The listing builds one solid part. Answer for the finished solid, in the listing's coordinates (mm). Face numbers are marked on the shaded views. A direction names the side the tool comes from. Coordinates: 2 decimals unless noted, no trailing zeros. Loops run counter-clockwise (first coordinate to the right, second up) from the corner with the lowest first, then second, coordinate; pieces in that order, holes last. Notation, with made-up numbers: (51, 24.25) -> (66, 24.25) arc R24 cw to (66, 53.25) -> close; hole circle Ø10 at (62, -1.75). An arc over 180 degrees is marked (long way). Answer in a Markdown table with one row per item.
Autodesk Inventor part; units mm, degrees
ref_plane "YZ Plane" through (0, 0, 0) normal (1, 0, 0) x (0, 1, 0)
ref_plane "XZ Plane" through (0, 0, 0) normal (0, 1, 0) x (-1, 0, 0)
ref_plane "XY Plane" through (0, 0, 0) normal (0, 0, 1) x (1, 0, 0)
sketch "Sketch1" plane through (0, 0, 0) normal (0, 0, 1) x (1, 0, 0)
  line L0 (4.1434, -12.66) -> (3.2904, -12.66)
  line L1 (-14.9, 12.8) -> (14.9, 12.8)
  line L2 (14.9, 12.8) -> (14.9, -12.8)
  line L3 (14.9, -12.8) -> (-14.9, -12.8)
  line L4 (-14.9, -12.8) -> (-14.9, 12.8)
  point P0 (0, 0)
  point P1 (0, 12.8)
  point P2 (-14.9, 0)
  dimension "d4" = 29.8
  dimension "d5" = 25.6
extrude "Extrusion1" add sketch "Sketch1" along normal blind 12.5
sketch "Sketch2" plane through (0, 0, 12.5) normal (0, 0, 1) x (1, 0, 0)
  line L0 (-14.9, -12.8) -> (14.9, -12.8)
  line L1 (-9.96, -12.8) -> (9.96, -12.8)
  line L2 (9.96, -12.8) -> (9.96, 7.8)
  line L3 (9.96, 7.8) -> (-9.96, 7.8)
  line L4 (-9.96, 7.8) -> (-9.96, -12.8)
  line L5 (14.9, 12.8) -> (-14.9, 12.8)
  point P0 (0, 0)
  point P1 (0, 7.8)
  dimension "d8" = 19.92
  dimension "d9" = 5
extrude "Extrusion2" cut sketch "Sketch2" against normal blind 7.5
sketch "Sketch3" plane through (0, 0, 12.5) normal (0, 0, 1) x (1, 0, 0)
  line L0 (-0.14, 0.6) -> (-0.84, 1.3)
  line L1 (14.9, -12.8) -> (14.9, 12.8)
  line L2 (14.9, -3.7) -> (26.6432, -3.7)
  line L3 (26.6432, -3.7) -> (26.6432, 12.8)
  line L4 (26.6432, 12.8) -> (14.9, 12.8)
  line L5 (14.9, 12.8) -> (14.9, -3.7)
  line L6 (14.9, 12.8) -> (-14.9, 12.8)
  line L7 (-7.482, 1.9485) -> (17.86, 10.1145)
  line L8 (-7.482, 1.9485) -> (19.1432, 1.9485)
  line L9 (9.96, 7.8) -> (9.96, -12.8)
  line L10 (9.96, 1.3) -> (21.6432, 1.3)
  line L11 (21.6432, 1.3) -> (21.6432, 7.8)
  line L12 (21.6432, 7.8) -> (9.96, 7.8)
  line L13 (9.96, 7.8) -> (9.96, 1.3)
  line L14 (-9.96, 7.8) -> (9.96, 7.8)
  point P0 (0, 0)
  point P1 (15.8016, 1.3)
  point P2 (21.6432, 4.55)
  dimension "d12" = 5
  dimension "d13" = 7.5
  dimension "d14" = 5
extrude "Extrusion3" add sketch "Sketch3" against normal blind 12.5 contours L1 L10 L11 L12 L4 L3 L2 | L1 L12 L11 L10
sketch "Sketch4" plane through (0, 0, 12.5) normal (0, 0, 1) x (1, 0, 0)
  line L0 (21.6432, 7.8) -> (9.96, 7.8)
  line L1 (9.96, 7.8) -> (9.96, 1.3)
  line L2 (9.96, 1.3) -> (21.6432, 1.3)
  line L3 (21.6432, 1.3) -> (21.6432, 7.8)
  point P0 (0, 0)
extrude "Extrusion4" cut sketch "Sketch4" against normal blind 7.5
thicken "Thicken1" operation add thickness 5 both sides no extend neighbours no toward (0, 1, 0) faces at (12.7954, 12.8, 4.1667)
sketch "Sketch5" plane through (0, 0, 12.5) normal (0, 0, 1) x (1, 0, 0)
  line L0 (-9.96, 7.8) -> (21.6432, 7.8)
  line L1 (-9.96, 7.8) -> (21.6432, 7.8)
  line L2 (21.6432, 7.8) -> (21.6432, 12.8)
  line L3 (21.6432, 12.8) -> (-9.96, 12.8)
  line L4 (-9.96, 12.8) -> (-9.96, 7.8)
  line L5 (21.6432, 7.8) -> (21.6432, 1.3)
  point P0 (0, 0)
  dimension "d21" = 5
extrude "Extrusion5" cut sketch "Sketch5" against normal blind 7.5
sketch "Sketch6" plane through (-14.9, -12.8, 0) normal (-1, 0, 0) x (0, 0, 1)
  circle A0 centre (8.2, 18.4735) radius 2.525
  line L0 (10, 14.7485) -> (6.4, 14.7485)
  line L1 (6.6, 15.3) -> (9.8, 15.3)
  point P0 (0, 12.8)
  point P1 (8.2, 14.7485)
  point P2 (8.2, 15.9485)
  dimension "d24" = 5.05
  dimension "d25" = 1.2
extrude "Extrusion6" cut sketch "Sketch6" against normal through all
properties part number "SS-5FL111-3T_Housing_01"
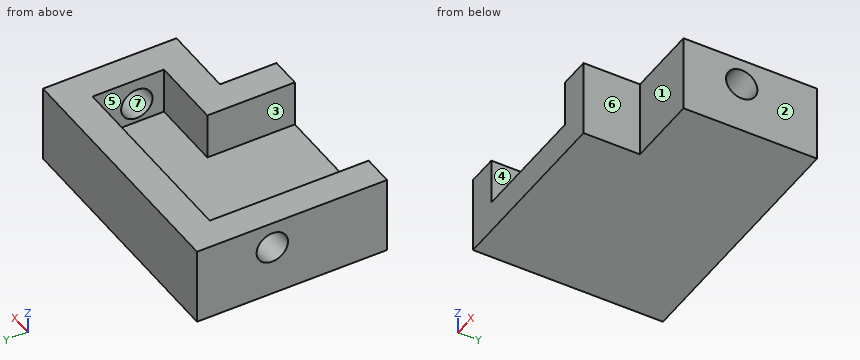
Item 1: A flat-ended cylindrical pin translates along its axis: pin 1 Ø6 at (x, y) = (15, 7.5) entering from +Z. Find the tip coordinate at first contact, or state that the pin passes through.
Findings below:
| item | result |
|---|---|
| pin 1 | stops at z = 5 |
Item 2: A tool of negligible diameter and unlimited length cuts with its end or side. For the marked faces 4, 5, 6 and 7, from which of +Z, -Z, +X, -X, +Y, -Y can it reach the whole face along a straight path? Write none if from no direction.
Findings below:
| item | result |
|---|---|
| face 4 | +Z, -Y |
| face 5 | +Z |
| face 6 | +Z, -Z, +X, -Y |
| face 7 | +X, -X |
Item 3: Find the intervals of material crossed by probe 1 along X at (y, z) = (-9.5, 5.5); probe 2 along Y at (x, z) = (-12.95, 8.2); probe 3 along Y at (x, z) = (24.85, 8.2), in increasing order.
Findings below:
| item | result |
|---|---|
| probe 1 | x = -14.9 to -9.96, 9.96 to 14.9 |
| probe 2 | y = -12.8 to 3.15, 8.2 to 17.8 |
| probe 3 | y = -3.7 to 3.15, 8.2 to 17.8 |
Item 4: Determine the mould class of the marked faces 1, 2 and 3 for opening direction X: +X half, -X half, draft (parallel to the pull), parting line (faces both ways), or undercut.
Findings below:
| item | result |
|---|---|
| face 1 | draft |
| face 2 | +X half |
| face 3 | undercut |
Item 5: A cutting plane is placed at B-B, the plane x = 19. Determine the outline of the cut face in (y, z), plus the area to 4 significant figures.
Findings below:
| item | result |
|---|---|
| outline | (-3.7, 0) -> (17.8, 0) -> (17.8, 12.5) -> (12.8, 12.5) -> (12.8, 5) -> (1.3, 5) -> (1.3, 12.5) -> (-3.7, 12.5) -> close |
| area | 182.5 mm2 |
Item 6: A cutting plane is placed at A-A, the plane z = 8.2. Determine the outline of the cut face in (x, y).
Findings below:
| item | result |
|---|---|
| outline | (-14.9, -12.8) -> (-9.96, -12.8) -> (-9.96, 3.15) -> (-14.9, 3.15) -> close; (-14.9, 8.2) -> (-9.96, 8.2) -> (-9.96, 12.8) -> (21.64, 12.8) -> (21.64, 8.2) -> (26.64, 8.2) -> (26.64, 17.8) -> (-14.9, 17.8) -> close; (9.96, -12.8) -> (14.9, -12.8) -> (14.9, -3.7) -> (26.64, -3.7) -> (26.64, 3.15) -> (21.64, 3.15) -> (21.64, 1.3) -> (9.96, 1.3) -> close |
Item 7: A cutting plane is placed at C-C, the plane y = -5. Determine the outline of the cut face in (x, z).
Findings below:
| item | result |
|---|---|
| outline | (-14.9, 0) -> (14.9, 0) -> (14.9, 12.5) -> (9.96, 12.5) -> (9.96, 5) -> (-9.96, 5) -> (-9.96, 12.5) -> (-14.9, 12.5) -> close |
